Job drawing, mm, ordinate dimensions from the low corner. One solid piece. Give positions to 0.01 mm unless a question says otherwise; leave off trailing zeros. Write each loop counter-clockwise with the first axis right and the second up, starting at its lowest first coordinate (ties: lowest second). Pieces come first, ordered by that corner, then holes. Notation, with made-up numbers: (12.5, 18) - (21.5, 18) arc R21 ccw to (21.5, 27) - close; hole circle Ø2 at (12, 87.5). An arc over 180 degrees is marked (long way). Answer in a Markdown table with one row per item. Add a question column.
1. Drop flat-ended pins along their axis: pin 1 Ø1.5 at (x, z) = (30, 27) entering from +Y; pin 2 Ø2 at (x, z) = (65.5, 30) entering from +Y; pin 3 Ø10 at (y, z) = (23, 38) entering from +X. Give the stop position or say it passes through.
2. Probe line 1 along Z through (x, y) = (63, 19); line 2 along Y through (x, z) = (66, 90) (1 decimal); line 3 along Y through (x, z) = (50.5, 52) (1 decimal). List the from-to ranges inside material, lowest first.
3. Band-saw the part on B-B on z = 16.5. Write the cut outline in (x, y) (1 decimal).
4. Band-saw the part on A-A on z = 114. Write the cut outline in (x, y) (1 decimal), plus the area to 3 significant figures.
5. Pull direction X, two halves, no side cores. Call the marked faces 1, 2 and 3: released by +X, released by -X, zero draft, split by the parting line, or undercut.
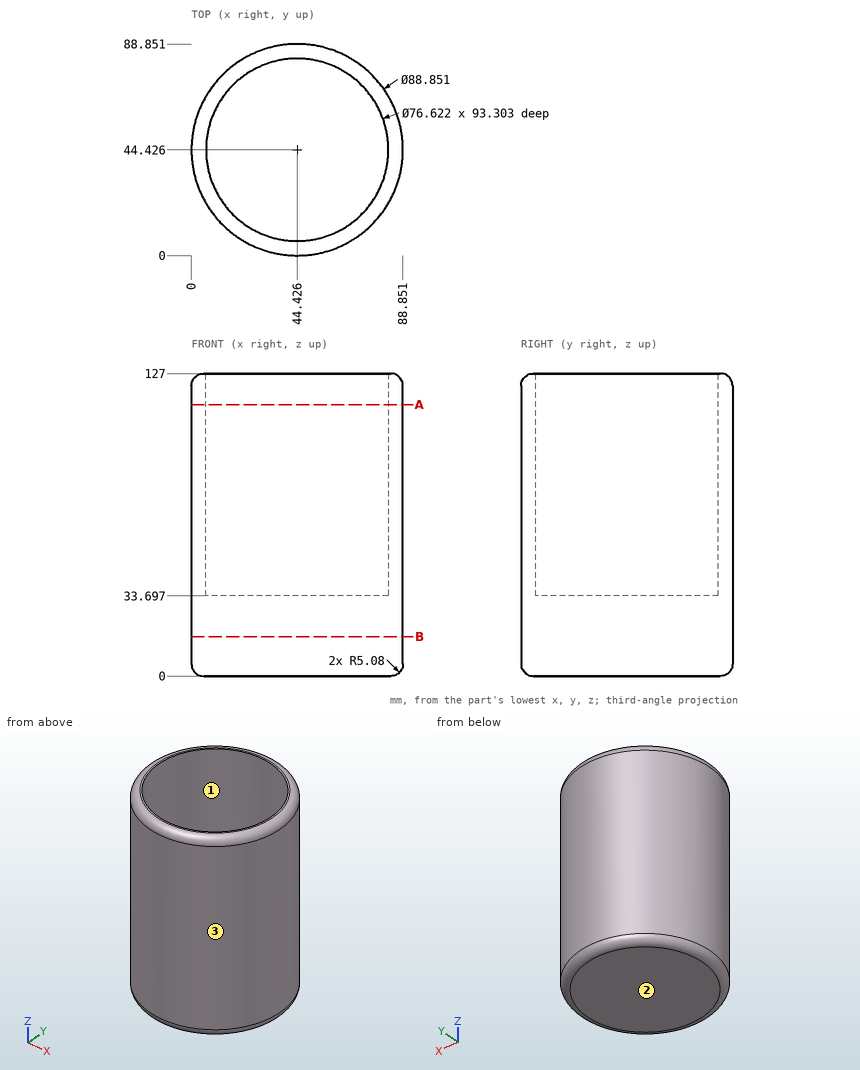
Values:
| question | item | result |
|---|---|---|
| 1 | pin 1 | stops at y = 86.69 |
| 1 | pin 2 | stops at y = 84.06 |
| 1 | pin 3 | stops at x = 85.7 |
| 2 | line 1 | z = 0 to 33.7 |
| 2 | line 2 | y = 5.6 to 12.8, 76.1 to 83.3 |
| 2 | line 3 | y = 0.4 to 6.6, 82.3 to 88.4 |
| 3 | outline | circle Ø88.9 at (44.4, 44.4) |
| 4 | outline | circle Ø88.9 at (44.4, 44.4); hole circle Ø76.6 at (44.4, 44.4) |
| 4 | area | 1,590 mm² |
| 5 | face 1 | undercut |
| 5 | face 2 | zero draft |
| 5 | face 3 | split by the parting line |
